Geometry: final body of the model. Coordinates: model frame, mm. A direction names the side the tool comes from. Give positions to 0.01 mm unless a question says otherwise; leave off trailing zeros. Write each loop counter-clockwise with the first axis right and the second up, starting at its lowest first coordinate (ties: lowest second). Pieces come first, ordered by that corner, then holes. Notation, with made-up numbers: (41.25, 34.25) -> (62.25, 34.25) arc R13 cw to (62.25, 48.25) -> close; hole circle Ø8 at (30.5, -40). An arc over 180 degrees is marked (long way). Answer in a Markdown table with one row per item. Add a question column.
from build123d import *
from OCP.BRepFilletAPI import BRepFilletAPI_MakeChamfer

# Parameters (mm, degrees)
SALIENTE_EXTRUIR1_DEPTH = 95
VACIADO1_T              = -5
CORTAR_EXTRUIR1_DEPTH   = 2.5
CROQUIS3_R              = 1.5
CORTAR_EXTRUIR4_DEPTH   = 5
SALIENTE_EXTRUIR2_DEPTH = 5
CHAFL_N1_SIZE           = 5
CHAFL_N1_SIZE2          = 1.819851171331016
CROQUIS5_R              = 1.5000000000000009
CORTAR_EXTRUIR5_DEPTH   = 107.86778586495213
CROQUIS6_W              = 80
CROQUIS6_H              = 6.500000000000014
CORTAR_EXTRUIR6_DEPTH   = 115.89125293076057
SALIENTE_EXTRUIR3_START = -5
SALIENTE_EXTRUIR3_DEPTH = 5
REDONDEO1_R             = 10
REDONDEO2_R             = 5
CROQUIS8_R              = 1.5000000000000004
CORTAR_EXTRUIR7_DEPTH   = 5


with BuildPart() as part:
    # Croquis1 → Saliente-Extruir1 (new body)
    with BuildSketch(Plane.XY):
        with BuildLine():
            Line((-40, 0), (40, 0))
            ThreePointArc((40, 0), (2.45e-15, 40), (-40, 0))
        make_face()
    extrude(amount=SALIENTE_EXTRUIR1_DEPTH)

    # Vaciado1
    vaciado1_openings = [part.faces().sort_by_distance(p)[0] for p in [
        (0, 16.976527263, 95),
        (0, 16.976527263, 0),
        (0, 0, 47.5),
    ]]
    offset(amount=VACIADO1_T, openings=vaciado1_openings)

    # Croquis2 → Cortar-Extruir1 (cut)
    with BuildSketch(Plane(origin=(0, 40, 0), x_dir=(1, 0, 0), z_dir=(0, 1, 0))):
        Polygon((2.499999999999998, 8), (-2.500000000000002, 8), (-2.499999999999997, -8), (2.500000000000003, -8), align=None)
    extrude(amount=-CORTAR_EXTRUIR1_DEPTH, mode=Mode.SUBTRACT)

    # Croquis3 → Cortar-Extruir4 (cut)
    with BuildSketch(Plane(origin=(0, 37.5, 0), x_dir=(1, 0, 0), z_dir=(0, 1, 0))):
        with Locations(Location((3.04e-15, -4.0000000000000036, 0), (0, 0, 270))):
            Circle(CROQUIS3_R)
    extrude(amount=-CORTAR_EXTRUIR4_DEPTH, mode=Mode.SUBTRACT)

    # Croquis4 → Saliente-Extruir2 (add, symmetric)
    with BuildSketch(Plane.XY.offset(95)):
        with BuildLine():
            Line((34.64101615137755, 20), (19.641016151377546, 20))
            Line((19.641016151377546, 20), (19.641016151377542, 9.999999999999998))
            Line((19.641016151377542, 9.999999999999998), (38.72983346207417, 10))
            ThreePointArc((38.72983346207417, 10), (37.024591736438325, 15.138679161342415), (34.64101615137755, 20))
        make_face()
        with BuildLine():
            Line((-19.641016151377542, 9.999999999999998), (-38.72983346207417, 10))
            ThreePointArc((-38.72983346207417, 10), (-37.024591736438325, 15.138679161342413), (-34.64101615137755, 20))
            Line((-34.64101615137755, 20), (-19.641016151377546, 20))
            Line((-19.641016151377546, 20), (-19.641016151377542, 9.999999999999998))
        make_face()
    extrude(amount=SALIENTE_EXTRUIR2_DEPTH, both=True)

    # Chaflán1: one chamfer whose edges measure the first distance from different faces: ONE call of the kernel's chamfer builder (chamfer() names one face for all edges)
    chafl_n1_edges_1 = [part.edges().sort_by_distance(p)[0] for p in [
        (27.14101615137755, 20, 100),
    ]]
    chafl_n1_side_1 = [part.faces().sort_by_distance(p)[0] for p in [
        (28.335600223521073, 14.80398786251226, 100),
    ]]
    chafl_n1_edges_2 = [part.edges().sort_by_distance(p)[0] for p in [
        (-27.14101615137755, 20, 100),
    ]]
    chafl_n1_side_2 = [part.faces().sort_by_distance(p)[0] for p in [
        (-28.33560022352108, 14.803987862512262, 100),
    ]]
    chafl_n1 = BRepFilletAPI_MakeChamfer(part.part.solid().wrapped)
    for e in chafl_n1_edges_1:
        chafl_n1.Add(CHAFL_N1_SIZE, CHAFL_N1_SIZE2, e.wrapped, chafl_n1_side_1[0].wrapped)  # the first distance lies on this face
    for e in chafl_n1_edges_2:
        chafl_n1.Add(CHAFL_N1_SIZE, CHAFL_N1_SIZE2, e.wrapped, chafl_n1_side_2[0].wrapped)  # the first distance lies on this face
    add(Compound.cast(chafl_n1.Shape()), mode=Mode.REPLACE)

    # Croquis5 → Cortar-Extruir5 (cut, through all)
    with BuildSketch(Plane(origin=(0, 33.89404716093429, 93.12312922859813), x_dir=(1, 0, 0), z_dir=(0, 0.3420201433256652, 0.9396926207859096))):
        with Locations(Location((-24.141016151377546, -17.446180589588106, 0), (0, 0, 270))):
            Circle(CROQUIS5_R)
        with Locations(Location((24.141016151377546, -17.446180589588106, 0), (0, 0, 90))):
            Circle(CROQUIS5_R)
    extrude(amount=-CORTAR_EXTRUIR5_DEPTH, mode=Mode.SUBTRACT)

    # Croquis6 → Cortar-Extruir6 (cut, through all)
    with BuildSketch(Plane(origin=(0, 0, 0), x_dir=(1, 0, 0), z_dir=(0, 1, 0))):
        with Locations((0, -98.25)):
            Rectangle(CROQUIS6_W, CROQUIS6_H)
    extrude(amount=CORTAR_EXTRUIR6_DEPTH, mode=Mode.SUBTRACT)

    # Croquis7 → Saliente-Extruir3 (add)
    with BuildSketch(Plane.XY.offset(95).offset(SALIENTE_EXTRUIR3_START)):
        with BuildLine():
            Line((19.641016151377542, 9.999999999999998), (35, 0))
            ThreePointArc((35, 0), (34.633334290733465, 5.052935375235389), (33.54101966249685, 10))
            Line((33.54101966249685, 10), (19.641016151377542, 9.999999999999998))
        make_face()
        with BuildLine():
            Line((-19.641016151377542, 9.999999999999998), (-35, 0))
            ThreePointArc((-35, 0), (-34.63333429073347, 5.0529353752354), (-33.54101966249685, 10))
            Line((-33.54101966249685, 10), (-19.641016151377542, 9.999999999999998))
        make_face()
        with BuildLine():
            Line((-19.641016151377546, 20), (-28.722813232690147, 20))
            ThreePointArc((-28.722813232690147, 20), (-26.75936830732511, 22.559614531124524), (-24.568594519878932, 24.927578368501326))
            Line((-24.568594519878932, 24.927578368501326), (-19.641016151377546, 20))
        make_face()
        with BuildLine():
            Line((19.641016151377546, 20), (28.722813232690147, 20))
            ThreePointArc((28.722813232690147, 20), (26.75936830732511, 22.559614531124524), (24.568594519878932, 24.927578368501326))
            Line((24.568594519878932, 24.927578368501326), (19.641016151377546, 20))
        make_face()
    extrude(amount=SALIENTE_EXTRUIR3_DEPTH)

    # Redondeo1
    redondeo1_edges = [part.edges().sort_by_distance(p)[0] for p in [
        (-19.641016151377546, 20, 92.5),
        (-19.641016151377542, 9.999999999999998, 92.5),
        (19.641016151377542, 9.999999999999998, 92.5),
        (19.641016151377546, 20, 92.5),
    ]]
    fillet(redondeo1_edges, radius=REDONDEO1_R)

    # Redondeo2
    # the kernel refuses this fillet: 5 mm, written as the material it adds along each edge
    with BuildSketch(Plane(origin=(24.568594519878932, 24.927578368501326, 90), x_dir=(-0.7663954409927094, 0.6423690746180039, 0), z_dir=(0, 0, 1))) as redondeo2_piece_1:
        with BuildLine():
            CenterArc((5.230741996241704, 4.983783963286785), REDONDEO2_R, 184.9379912398929, 89.6777604033997)
            Line((0.2492997983567551, 4.553396197276695), (-0.24884442143173913, 4.510357420675686))
            ThreePointArc((-0.24884442143173913, 4.510357420675686), (-0.2501886476220602, 2.859471760516391), (-0.4980734710416599, 0.04384994235474339))
            Line((-0.4980734710416599, 0.04384994235474339), (-0.04023647689416843, -0.49837839632867914))
            ThreePointArc((-0.04023647689416843, -0.49837839632867914), (2.816553382591687, -0.6135122569925113), (5.673343242077539, -0.49837839632867886))
            Line((5.673343242077539, -0.49837839632867886), (5.633106765183373, 2.3e-16))
        make_face()
    extrude(amount=5)
    with BuildSketch(Plane(origin=(-24.568594519878932, 24.927578368501326, 90), x_dir=(0.7663954409927088, 0.6423690746180043, 0), z_dir=(0, 0, 1))) as redondeo2_piece_2:
        with BuildLine():
            CenterArc((5.2307419962416954, -4.9837839632867835), REDONDEO2_R, 85.38424835670739, 89.67776040339973)
            Line((0.24929979835674423, -4.553396197276693), (-0.24884442143174967, -4.510357420675684))
            ThreePointArc((-0.24884442143174967, -4.510357420675684), (-0.2501886476220599, -2.8594717605163877), (-0.4980734710416599, -0.04384994235474303))
            Line((-0.4980734710416599, -0.04384994235474303), (-0.0402364768941681, 0.4983783963286791))
            ThreePointArc((-0.0402364768941681, 0.4983783963286791), (2.816553382591687, 0.6135122569925143), (5.673343242077529, 0.49837839632867875))
            Line((5.673343242077529, 0.49837839632867875), (5.633106765183362, 3.7e-16))
        make_face()
    extrude(amount=5)

    # Croquis8 → Cortar-Extruir7 (cut)
    with BuildSketch(Plane.XY.offset(95)):
        with Locations((2.3e-15, 37.50000000000001)):
            Circle(CROQUIS8_R)
    extrude(amount=-CORTAR_EXTRUIR7_DEPTH, mode=Mode.SUBTRACT)


solid = part.part
Q1. Section D-D on z = 58. Return loops of the section in (x, y).
Q2. Contact query for flat-ended pins moving along their axis: pin 1 Ø2 at (y, z) = (5, 10.5) entering from -X; pin 2 Ø1 at (x, z) = (-3.5, 54.5) entering from -Y; pin 3 Ø2 at (x, z) = (21, 42.5) entering from -Y. Output: stop coordinate, or through.
Q3. Pull-direction query (Z, two-part tool) for faces 5 (the flat face through (4, 35, 95)), 6 (the cylindrical face through (23.69, 16.453, 92.029)), 7 (the flat face through (-2.5, 39, 4)), 8 (the cylindrical face through (-24.075, 16.534, 92.054)); classes: +Z half, -Z half, draft (parallel to the pull), parting line (faces both ways), or undercut.
Q4. Section B-B on x = 0. Return loops of the section in (y, z).
Q5. Section C-C on y = 4. Return loops of the section in (x, z), and give its area (3 significant figures).
Q6. Access query for faces 1 (the cylindrical face through (-22.276, 25.374, 92.465)), 2 (the flat face through (0, 38, 90)), 3 (the flat face through (0, 39, 8)), 4 (the cylindrical face through (20.883, 10.594, 92.535)). Directions: +Z, -Z, +X, -X, +Y, -Y. A direction counts if a zero-diameter tool reaches every point of the face in a straight line with its end or side. Return the directions, or none.
Q7. Line query: probe 1 along X at (y, z) = (37, 93); probe 2 along Z at (x, y) = (-34.5, 3); probe 3 along X at (y, z) = (9.5, 89.5). Output: solid intervals per line, ascending. Write a range as from..to.
Checks:
| question | item | result |
|---|---|---|
| 1 | outline | (-40, 0) -> (-35, 0) arc R35 cw to (35, 0) -> (40, 0) arc R40 ccw to start |
| 2 | pin 1 | x = -39.8 |
| 2 | pin 2 | y = 34.77 |
| 2 | pin 3 | y = 27.22 |
| 3 | face 5 | +Z half |
| 3 | face 6 | undercut |
| 3 | face 7 | draft |
| 3 | face 8 | undercut |
| 4 | outline | (35, 0) -> (37.5, 0) -> (37.5, 2.5) -> (35, 2.5) -> close; (35, 5.5) -> (37.5, 5.5) -> (37.5, 8) -> (40, 8) -> (40, 95) -> (39, 95) -> (39, 90) -> (36, 90) -> (36, 95) -> (35, 95) -> close |
| 5 | outline | (-39.8, 0) -> (-34.77, 0) -> (-34.77, 90) -> (-28.86, 90) -> (-28.86, 95) -> (-39.8, 95) -> close; (28.86, 90) -> (34.77, 90) -> (34.77, 0) -> (39.8, 0) -> (39.8, 95) -> (28.86, 95) -> close |
| 5 | area | 1,010 mm^2 |
| 6 | face 1 | +Z, -Z |
| 6 | face 2 | +Z |
| 6 | face 3 | -Z, +Y |
| 6 | face 4 | +Z, -Z, -Y |
| 7 | probe 1 | -15.2..-1.41, 1.41..15.2 |
| 7 | probe 2 | 90..95 |
| 7 | probe 3 | -38.86..-33.69, 33.69..38.86 |
